Source: CAD feature listing. Evaluate the final solid. Frame: model axes, mm. A direction names the side the tool comes from. Give positions to 0.01 mm unless a question says otherwise; leave off trailing zeros. Write each loop counter-clockwise with the first axis right and the second up, starting at its lowest first coordinate (ties: lowest second). Pieces come first, ordered by that corner, then holes. Notation, with made-up numbers: (18.25, 58) - (60.25, 58) arc R31 cw to (60.25, 85) - close; hole circle Ø10 at (-31, 24.25). An arc over 180 degrees is marked (long way). One line per question, with ' | ' between items. Start each with the question number.
(1) Section B-B, the plane x = -1. Return loops of the section in (y, z).
(2) Access query for faces 1 (the flat face through (10, -24, 1)), 2 (the flat face through (-55.5, 0, 1)), 3 (the flat face through (-37, -22.5, 1)), 4 (the flat face through (-49, 22.5, 1)). Directions: +Z, -Z, +X, -X, +Y, -Y. A direction counts if a zero-diameter tool reaches every point of the face in a straight line with its end or side. Return the directions, or none.
(3) Pin query (flat end, axial travel): pin 1 (1.5 mm diameter, centred on x = 34, z = 1, fed in from -Y); pin 2 (1.5 mm diameter, centred on y = 0, z = 1.5, fed in from -X). Return the tip coordinate at first contact, or that it passes through.
(4) Section C-C, the plane z = 2.5. State how many separate pieces and enclosed holes the cut face has, plus the area to 3 significant figures.
(5) Draft query along Y for faces 5 (the flat face through (-64, -10, 1)), 6 (the flat face through (49, 22.5, 1)), 7 (the flat face through (1, -5, 0)). Return one class per face: +Y half, -Y half, draft (parallel to the pull), parting line (faces both ways), or undercut.
(6) Ray query, line 1 (X direction, y = 5, z = 0.3); line 2 (Y direction, x = 10.75, z = 1.8); line 3 (Y direction, x = 0, z = 2.3). Return the intervals inside material, ascending. Write a range as [from, to].
(7) Section A-A, the plane x = -48.5. Return loops of the section in (y, z), plus the area to 3 significant figures.
(8) Section D-D, the plane x = -27. Return loops of the section in (y, z), plus the area to 3 significant figures.
```python
from build123d import *

# Parameters (mm, degrees)
SKETCH1_R           = 9.25
SKETCH1_R_2         = 4.5
SKETCH1_R_3         = 2.5
SKETCH1_R_4         = 1.25
BOSS_EXTRUDE1_DEPTH = 3


with BuildPart() as part:
    # Sketch1 → Boss-Extrude1 (new body)
    with BuildSketch(Plane.XY):
        Polygon((-10, -22.5), (-65, -22.5), (-65, -10), (-62, -10), (-62, 10), (-65, 10), (-65, 22.5), (-33.3, 22.5), (-33.3, 19.5), (-34.65, 19.5), (-34.65, 17), (-33.3, 17), (-33.3, 12.5), (-30, 12.5), (-30, 17), (-28.65, 17), (-28.65, 19.5), (-30, 19.5), (-30, 22.5), (-10, 22.5), (-10, 25.5), (10, 25.5), (10, 22.5), (30, 22.5), (30, 19.5), (28.65, 19.5), (28.65, 17), (30, 17), (30, 12.5), (33.3, 12.5), (33.3, 17), (34.65, 17), (34.65, 19.5), (33.3, 19.5), (33.3, 22.5), (65, 22.5), (65, 10), (62, 10), (62, -10), (65, -10), (65, -22.5), (10, -22.5), (10, -25.5), (-10, -25.5), align=None)
        with Locations((-49.5, 12.75)):
            Circle(SKETCH1_R, mode=Mode.SUBTRACT)
        with Locations((-49.5, -12.75)):
            Circle(SKETCH1_R, mode=Mode.SUBTRACT)
        Circle(SKETCH1_R_2, mode=Mode.SUBTRACT)
        with Locations((10.75, 0)):
            Circle(SKETCH1_R_3, mode=Mode.SUBTRACT)
        with Locations((-9, 9.25)):
            Circle(SKETCH1_R_4, mode=Mode.SUBTRACT)
        with Locations(Location((-9, -9.25, 0), (0, 0, 180))):
            Circle(SKETCH1_R_4, mode=Mode.SUBTRACT)
        with BuildLine():
            Line((-55.5, 3.5), (-55.5, -3.5))
            ThreePointArc((-55.5, -3.5), (-58, -6), (-60.5, -3.5))
            Line((-60.5, -3.5), (-60.5, 3.5))
            ThreePointArc((-60.5, 3.5), (-58, 6), (-55.5, 3.5))
        make_face(mode=Mode.SUBTRACT)
        with BuildLine():
            Line((-40.5, -6), (-41.5, -6))
            ThreePointArc((-41.5, -6), (-42.914213562, -5.414213562), (-43.5, -4))
            Line((-43.5, -4), (-43.5, 4))
            ThreePointArc((-43.5, 4), (-42.914213562, 5.414213562), (-41.5, 6))
            Line((-41.5, 6), (-40.5, 6))
            Line((-40.5, 6), (-40.5, -6))
        make_face(mode=Mode.SUBTRACT)
        with BuildLine():
            Line((39, -5), (39, 5))
            ThreePointArc((39, 5), (47, 13), (55, 5))
            Line((55, 5), (55, -5))
            ThreePointArc((55, -5), (47, -13), (39, -5))
        make_face(mode=Mode.SUBTRACT)
    extrude(amount=BOSS_EXTRUDE1_DEPTH)


solid = part.part
```
Check sheet entries:
1) outline: (-25.5, 0) - (-4.39, 0) - (-4.39, 3) - (-25.5, 3) - close; (4.39, 0) - (25.5, 0) - (25.5, 3) - (4.39, 3) - close
2) face 1: +Z, -Z, +X, -Y | face 2: +Z, -Z | face 3: +Z, -Z, -X, -Y | face 4: +Z, -Z, -X, +Y
3) pin 1: y = -22.5 | pin 2: x = -62
4) separate pieces: 1 | enclosed holes: 9 | area: 4,690 mm²
5) face 5: undercut | face 6: +Y half | face 7: draft
6) line 1: [-62, -60], [-56, -54.55], [-44.45, -43.23], [-40.5, 39], [55, 62] | line 2: [-22.5, -2.5], [2.5, 22.5] | line 3: [-25.5, -4.5], [4.5, 25.5]
7) outline: (-22.5, 0) - (-21.95, 0) - (-21.95, 3) - (-22.5, 3) - close; (-3.55, 0) - (3.55, 0) - (3.55, 3) - (-3.55, 3) - close; (21.95, 0) - (22.5, 0) - (22.5, 3) - (21.95, 3) - close | area: 24.7 mm²
8) outline: (-22.5, 0) - (22.5, 0) - (22.5, 3) - (-22.5, 3) - close | area: 135 mm²
